The model under review builds one solid part; all positions refer to its coordinate system, in mm. A direction names the side the tool comes from. Give positions to 0.01 mm unless a question says otherwise; leave off trailing zeros. Write each loop counter-clockwise with the first axis right and the second up, starting at its lowest first coordinate (ties: lowest second). Pieces come first, ordered by that corner, then holes. Notation, with made-up numbers: (63.5, 47) - (108.5, 47) arc R9 ccw to (108.5, 51) - close; hole circle Ø9 at (-4, 86.25). An arc over 180 degrees is marked (long way). Write item = value, one per line.
```python
from build123d import *

# Parameters (mm, degrees)
F0_W      = 38.1832793355
F0_H      = 63.5416381992
F1_DEPTH  = 5.842
F2_R      = 5.08
F3_W      = 38.1832793355
F3_H      = 51.7094545066
F4_DEPTH  = 19.05
F5_W      = 19.0890878439
F5_H      = 41.4883207995
F6_DEPTH  = 19.05
F8_R      = 13.8442198494
F9_DEPTH  = 25.4
F10_W     = 12.3838447034
F10_H     = 8.160058409
F11_DEPTH = 19.05


with BuildPart() as f1:
    # F0 (on Top) → F1 (new body)
    with BuildSketch(Plane.XY):
        with Locations((-39.9321317673, 24.1924587172)):
            Rectangle(F0_W, F0_H)
    extrude(amount=F1_DEPTH)

    # F2
    f2_edges = [f1.edges().sort_by_distance(p)[0] for p in [
        (-59.023771, 55.963278, 2.921),
        (-59.023771, -7.57836, 2.921),
    ]]
    fillet(f2_edges, radius=F2_R)

    # F3 (on face) → F4 (join)
    with BuildSketch(Plane.XY.offset(5.842)):
        with Locations((-39.9321317673, 22.9528117925)):
            Rectangle(F3_W, F3_H)
    extrude(amount=F4_DEPTH)

    # F5 (on face) → F6 (cut)
    with BuildSketch(Plane.XY.offset(24.892)):
        with Locations((-30.3850360215, 23.5381604871)):
            Rectangle(F5_W, F5_H)
    extrude(amount=-F6_DEPTH, mode=Mode.SUBTRACT)

    # F8 (on face) → F9 (cut)
    with BuildSketch(Plane.XY.offset(24.892)):
        with Locations((-58.3629384637, 23.0822730809)):
            Circle(F8_R)
    extrude(amount=-F9_DEPTH, mode=Mode.SUBTRACT)

    # F10 (on face) → F11 (cut)
    with BuildSketch(Plane.XY.offset(24.892)):
        with Locations((-52.489342168, 44.8476765305)):
            Rectangle(F10_W, F10_H)
    extrude(amount=-F11_DEPTH, mode=Mode.SUBTRACT)


solid = f1.part
```
1. Take a section at D-D on y = 3.5. Give the boundary of the cut face in (x, z).
Findings below:
outline = (-59.02, 0) - (-20.84, 0) - (-20.84, 5.84) - (-39.93, 5.84) - (-39.93, 24.89) - (-59.02, 24.89) - close
2. Take a section at A-A on y = 41.5. Give the boundary of the cut face in (x, z).
Findings below:
outline = (-59.02, 0) - (-20.84, 0) - (-20.84, 5.84) - (-39.93, 5.84) - (-39.93, 24.89) - (-46.3, 24.89) - (-46.3, 5.84) - (-58.68, 5.84) - (-58.68, 24.89) - (-59.02, 24.89) - close
3. Take a section at C-C on z = 10.5. Give the boundary of the cut face in (x, y).
Findings below:
outline = (-59.02, -2.9) - (-20.84, -2.9) - (-20.84, 2.79) - (-39.93, 2.79) - (-39.93, 44.28) - (-20.84, 44.28) - (-20.84, 48.81) - (-46.3, 48.81) - (-46.3, 40.77) - (-58.68, 40.77) - (-58.68, 48.81) - (-59.02, 48.81) - (-59.02, 36.91) arc R13.84 cw (long way) to (-59.02, 9.25) - close
4. For line 1 (Y direction, x = -33, z = 12.5); line 2 (Z direction, x = -52, y = 46); line 3 (X direction, y = 5, z = 10), list the stretches that pass through material, from the lowest coordinate up. Write a range as from..to.
Findings below:
line_1 = -2.9..2.79, 44.28..48.81
line_2 = 0..5.84
line_3 = -59.02..-39.93
5. Draft analysis for pull direction Y (two halves, no side actions). For faces 1 (the flat face through (-20.84, 24, 4)), 2 (the flat face through (-38, 55.963, 3)), 3 (the flat face through (-39.93, 23, 16)), state which applies: +Y half, -Y half, draft (parallel to the pull), parting line (faces both ways), or undercut.
Findings below:
face_1 = draft
face_2 = +Y half
face_3 = undercut
6. Take a section at B-B on x = -32. Give the boundary of the cut face in (y, z), and give its area (3 significant figures).
Findings below:
outline = (-7.58, 0) - (55.96, 0) - (55.96, 5.84) - (48.81, 5.84) - (48.81, 24.89) - (44.28, 24.89) - (44.28, 5.84) - (2.79, 5.84) - (2.79, 24.89) - (-2.9, 24.89) - (-2.9, 5.84) - (-7.58, 5.84) - close
area = 566 mm²
7. Insertion check: P1, Ø5.5, axis at x = -29, z = 13, coming from the +Y side; P2, Ø5.5, axis at x = -33.5, z = 10.5, coming from the -Y side; P3, Ø1.5, axis at y = 19, z = 7.5, coming from the +X side. Each pin has a flat end and moves straight along its axis. Give the tip position at first contact, or say it passes through.
Findings below:
P1 = 48.81
P2 = -2.9
P3 = -39.93
8. Machinability: for faces 4 (the flat face through (-31, 44.282, 16)), 5 (the flat face through (-58.681, 45, 16)), 6 (the flat face through (-34, 48.808, 15)), which of the approach directions +Z, -Z, +X, -X, +Y, -Y give a long, thin tool a straight path to every point of the face, cutting with its end or side? Answer none if there is none.
Findings below:
face_4 = +Z, +X
face_5 = +Z, +Y
face_6 = +Z, +X, -X, +Y
